Design review of the part shown in the three views and the two pictorial views. Dimensions are in mm from the part's minimum x, y and z. A direction names the side the tool comes from. Round coordinates to 2 decimals unless told otherwise and drop trailing zeros. Write each loop counter-clockwise with the first axis right and the second up, starting at its lowest first coordinate (ties: lowest second). Pieces come first, ordered by that corner, then holes. Notation, with made-up numbers: (-9.75, 52.25) -> (41.25, 52.25) arc R31 ccw to (41.25, 78.25) -> close; hole circle Ø10 at (86, 88.5). An arc over 180 degrees is marked (long way). Return JSON: item names as keys, results as strings. Group by question number.
1. Take a section at A-A, the plane x = 108. Write out the cut boundary in (y, z), then the cut area to 3 significant figures.
2. For line 1 along Y through (x, z) = (97, 16); line 2 along Z through (x, y) = (10, 5); line 3 along Y through (x, z) = (129.5, 27.5) (1 decimal), list the stretches that pass through material, from the lowest coordinate up. Write a range as from..to.
3. Take a section at C-C, the plane y = 4.25. Write out the cut boundary in (x, z).
4. Take a section at B-B, the plane z = 15. Write out the cut boundary in (x, y), then the cut area to 3 significant figures.
5. Clearance check with flat-ended pins moving along their axes: P1, Ø4, axis at x = 19.78, y = 13.29, coming from the -Z side; P2, Ø10, axis at x = 50, y = 4, coming from the -Z side; P3, Ø1.5, axis at x = 108, z = 22.5, coming from the -Y side; P4, Ø12, axis at y = 9, z = 17, coming from the -X side. State where each tip first meets the part, or that it passes through.
6. Tool access review of the marked faces 1 and 2: name each direction out of +Z, -Z, +X, -X, +Y, -Y from which nothing blocks a thin tool from reaching the whole face with its end or side.
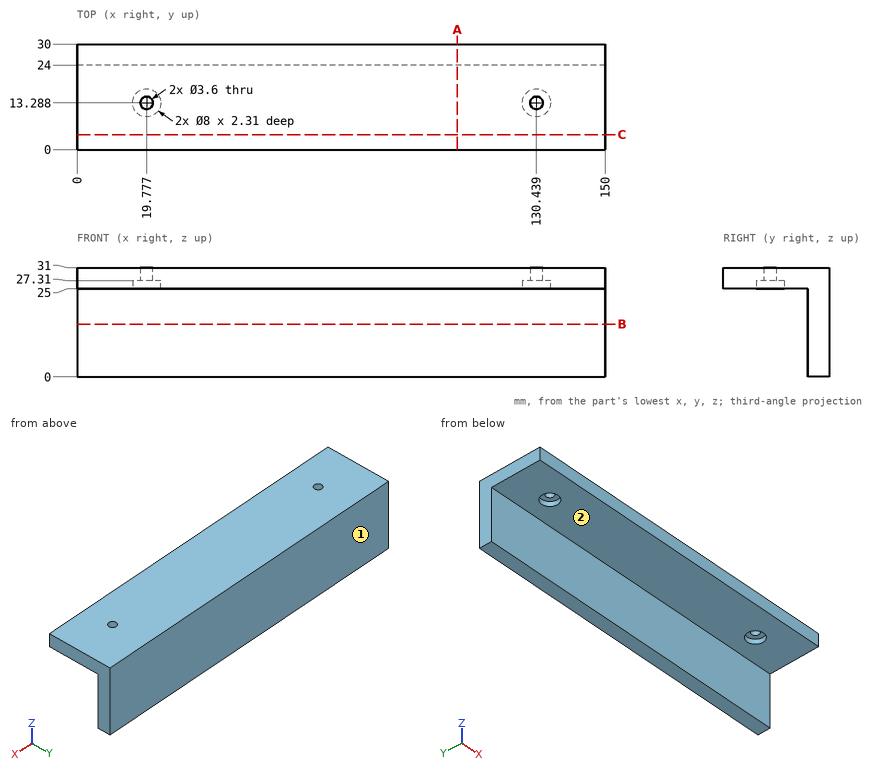
Output:
{
 "1": {"outline": "(0, 25) -> (24, 25) -> (24, 0) -> (30, 0) -> (30, 31) -> (0, 31) -> close", "area": "330 mm^2"},
 "2": {"line 1": "y = 24..30", "line 2": "z = 25..31", "line 3": "y = 0..11.8, 14.8..30"},
 "3": {"outline": "(0, 25) -> (150, 25) -> (150, 31) -> (0, 31) -> close"},
 "4": {"outline": "(0, 24) -> (150, 24) -> (150, 30) -> (0, 30) -> close", "area": "900 mm^2"},
 "5": {"P1": "stops at z = 27.31", "P2": "stops at z = 25", "P3": "stops at y = 24", "P4": "passes through"},
 "6": {"face 1": "+Z, -Z, +X, -X, +Y", "face 2": "-Z, +X, -X, -Y"}
}
